Verification items for the finished model (mm, model axes). Face numbers are marked on the shaded views. A direction names the side the tool comes from. Coordinates: 2 decimals unless noted, no trailing zeros. Order: outer loops, then holes, each group sorted by start corner. A loop starts at its lowest first (then second) coordinate and runs counter-clockwise, first axis right, second up. Notation, with made-up numbers: M 50,-19 L 79,-19 A16 cw 79,-7 Z; hole C -30.75,35.25 d6. An arc over 180 degrees is marked long. Return JSON: item names as keys, results as strings. Group by question number.
Q1. Access from +Z, -Z, +X, -X, +Y, -Y to the whole of each face (thin tool, end or side, straight path). Record for the marked faces 1, 2 and 3.
Q2. Section check C-C, the plane y = 47.5. Enter the section's corners in (x, z), then the cut area to 3 significant figures.
Q3. Thickness scan on probe 1 along Y at (x, z) = (0.5, 2.25); probe 2 along X at (y, z) = (49.5, -0.25); probe 3 along Y at (x, z) = (-11.5, 0.25). Record the ranges inside material, lowest first.
Q4. Section check A-A, the plane x = 0. Enter the section's corners in (y, z), then the cut area to 3 significant figures.
Q5. Go/stop test with flat-tipped pins: pin 1 Ø5.5 at (x, z) = (0.5, 0.5) entering from +Y; pin 2 Ø5 at (y, z) = (41, 6.5) entering from +X; pin 3 Ø5 at (y, z) = (27, 6) entering from +X; pin 4 Ø3 at (x, y) = (-1.5, 50) entering from +Z. Record where each tip stops, or that it passes through.
Q6. Mould release check, pull along X, two halves, no side actions. Record for the marked faces 4, 5 and 6: pulls with the +X half, pulls with the -X half, needs draft (parallel to the pull), parting line crosses it, or undercut.
Q7. Section check B-B, the plane z = 0. Enter the section's corners in (x, y), then the cut area to 3 significant figures.
from build123d import *

# Parameters (mm, degrees)
EXTRUDE_START       = 15
SKETCH_1_R          = 10
EXTRUDE_1_DEPTH     = 40.4
SKETCH_2_R          = 3.5
CUT_EXTRUDE_1_DEPTH = 34
SKETCH_3_R          = 12.7
EXTRUDE_2_DEPTH     = 4
FILLET_4_R          = 0.5


with BuildPart() as part:
    # Эскиз1 → Вытянуть1 (new body)
    with BuildSketch(Plane(origin=(0, 0, 0), x_dir=(1, 0, 0), z_dir=(0, 1, 0)).offset(EXTRUDE_START)):
        with Locations(Location((0, 0, 0), (0, 0, 270))):
            Circle(SKETCH_1_R)
    extrude(amount=EXTRUDE_1_DEPTH)

    # Эскиз2 → Вырез-Вытянуть1 (cut)
    with BuildSketch(Plane(origin=(0, 55.4, 0), x_dir=(1, 0, 0), z_dir=(0, 1, 0))):
        with Locations(Location((0, 0, 0), (0, 0, 270))):
            Circle(SKETCH_2_R)
    extrude(amount=-CUT_EXTRUDE_1_DEPTH, mode=Mode.SUBTRACT)

    # Эскиз3 → Вытянуть2 (add)
    with BuildSketch(Plane(origin=(0, 52.4, 0), x_dir=(-1, 0, 0), z_dir=(0, 1, 0))):
        with Locations(Location((0, 0, 0), (0, 0, 90))):
            Circle(SKETCH_3_R)
    extrude(amount=-EXTRUDE_2_DEPTH)

    # Скругление4
    fillet_4_edges = [part.edges().sort_by_distance(p)[0] for p in [
        (0, 52.4, -12.7),
        (0, 48.4, -12.7),
    ]]
    fillet(fillet_4_edges, radius=FILLET_4_R)


solid = part.part
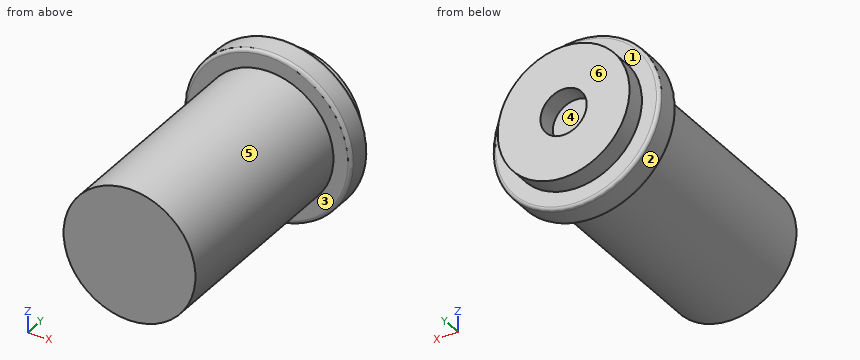
Numbers:
{
 "1": {"face 1": "+Y", "face 2": "+Y, -Y", "face 3": "-Y"},
 "2": {"outline": "C 0,0 d20; hole C 0,0 d7", "area": "276 mm2"},
 "3": {"probe 1": "y = 15 to 21.4, 48.4 to 52.4", "probe 2": "x = -12.7 to 12.7", "probe 3": "y = 48.4 to 52.4"},
 "4": {"outline": "M 15,-10 L 48.4,-10 L 48.4,-12.2 A0.5 ccw 48.9,-12.7 L 51.9,-12.7 A0.5 ccw 52.4,-12.2 L 52.4,-10 L 55.4,-10 L 55.4,-3.5 L 52.4,-3.5 L 52.4,3.5 L 55.4,3.5 L 55.4,10 L 52.4,10 L 52.4,12.2 A0.5 ccw 51.9,12.7 L 48.9,12.7 A0.5 ccw 48.4,12.2 L 48.4,10 L 15,10 Z; hole M 21.4,-3.5 L 48.4,-3.5 L 48.4,3.5 L 21.4,3.5 Z", "area": "619 mm2"},
 "5": {"pin 1": "stops at y = 52.4", "pin 2": "stops at x = 9.17", "pin 3": "stops at x = 9.37", "pin 4": "stops at z = 12.7"},
 "6": {"face 4": "undercut", "face 5": "parting line crosses it", "face 6": "needs draft"},
 "7": {"outline": "M -12.7,48.9 A0.5 ccw -12.2,48.4 L -10,48.4 L -10,15 L 10,15 L 10,48.4 L 12.2,48.4 A0.5 ccw 12.7,48.9 L 12.7,51.9 A0.5 ccw 12.2,52.4 L 10,52.4 L 10,55.4 L 3.5,55.4 L 3.5,52.4 L -3.5,52.4 L -3.5,55.4 L -10,55.4 L -10,52.4 L -12.2,52.4 A0.5 ccw -12.7,51.9 Z; hole M -3.5,21.4 L 3.5,21.4 L 3.5,48.4 L -3.5,48.4 Z", "area": "619 mm2"}
}
